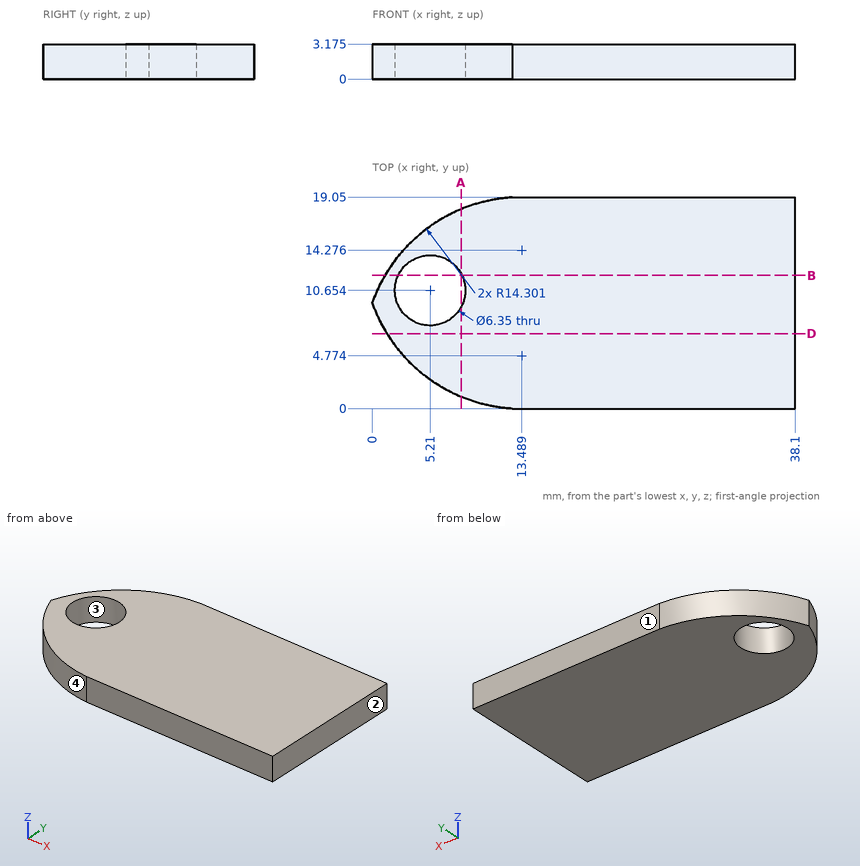
Verification items for this drawing (mm, ordinates from the low corner). Give positions to 0.01 mm unless a question says otherwise; leave off trailing zeros. Write each loop counter-clockwise with the first axis right and the second up, starting at its lowest first coordinate (ties: lowest second). Pieces come first, ordered by that corner, then holes.
1) Section check D-D, the plane y = 6.75. Record the boundary of the cut face in (x, z) (1 decimal), and give its area (3 significant figures).
2) Gauge pin test, flat end, axial feed: pin 1 (1.5 mm diameter, centred on y = 12.5, z = 1.5, fed in from -X) (1 decimal). Record the tip position at first contact, or that the pin passes through.
3) Material ranges on L1, parallel to X at y = 13.5, z = 2.4 (1 decimal); L2, parallel to X at y = 9.5, z = 2.05; L3, parallel to X at y = 15.5, z = 2.5, recorded low to high.
4) Section check A-A, the plane x = 8. Record the boundary of the cut face in (y, z) (1 decimal).
5) Release check for a two-part mould opening along Y. For the marked faces 1, 2, 3 and 4 record: pulls with the +Y half, pulls with the -Y half, needs draft (parallel to the pull), parting line crosses it, or undercut.
6) Section check B-B, the plane y = 12. Record the boundary of the cut face in (x, z) (1 decimal).
Computed:
1. outline: (1.3, 0) - (38.1, 0) - (38.1, 3.2) - (1.3, 3.2) - close
1. area: 117 mm2
2. pin 1: stops at x = 1
3. L1: x = 2.2 to 3.8, 6.6 to 38.1
3. L2: x = 0.01 to 2.25, 8.17 to 38.1
3. L3: x = 4.03 to 38.1
4. outline: (1.1, 0) - (9.1, 0) - (9.1, 3.2) - (1.1, 3.2) - close; (12.2, 0) - (18, 0) - (18, 3.2) - (12.2, 3.2) - close
5. face 1: pulls with the +Y half
5. face 2: needs draft
5. face 3: undercut
5. face 4: pulls with the -Y half
6. outline: (1.1, 0) - (2.3, 0) - (2.3, 3.2) - (1.1, 3.2) - close; (8.1, 0) - (38.1, 0) - (38.1, 3.2) - (8.1, 3.2) - close
